Can you work these out from the drawing? Everything is in mm from the part's minimum corner. A direction names the side the tool comes from. Coordinates: 2 decimals unless noted, no trailing zeros. Order: outer loops, then holes, each group sorted by start corner. A loop starts at its lowest first (then second) coordinate and runs counter-clockwise, first axis right, second up. Notation, with made-up numbers: (84, 62) - (126, 62) arc R23 ccw to (126, 79) - close; hole circle Ø2 at (13.25, 88). An arc over 180 degrees is marked (long way). Answer as CSV lines item,"result". Start each with the question number.
Item 1: I'm going to push flat-ended pins straight in: pin 1 (2 mm diameter, centred on y = 9.5, z = 15, fed in from +X); pin 2 (4 mm diameter, centred on x = 11.5, y = 3.5, fed in from +Z); pin 3 (5 mm diameter, centred on x = 13, z = 3, fed in from +Y). Where does each tip first touch, or does it pass through?
Item 2: Imagine slicing it at B-B on z = 9.25. List the corners of the cut face in (x, y) for me.
Item 3: We'd pull the mould along X, two halves only. Please class the marked faces 6, 7 and 8: pulls with the +X half, pulls with the -X half, needs draft (parallel to the pull), parting line crosses it, or undercut.
Item 4: Imagine slicing it at D-D on y = 8. List the corners of the cut face in (x, z) for me, and give its area (3 significant figures).
Item 5: On a 3-axis mill with a long thin cutter (end or side, diameter ignored), from which of +Z, -Z, +X, -X, +Y, -Y can I reach the whole of each face in a straight line? I mean the marked faces 1, 2, 3, 4 and 5. Say none if no direction works.
Item 6: I need wall thicknesses on line 1 (X direction, y = 12.75, z = 8.5); line 2 (Z direction, x = 22.25, y = 1.75). Which ranges of each line are inside material? Lowest first, please.
Item 7: Imagine slicing it at C-C on x = 14. List the corners of the cut face in (y, z) for me, and give its area (3 significant figures).
Item 8: Imagine slicing it at A-A on y = 15. List the corners of the cut face in (x, z) for me, and give its area (3 significant figures).
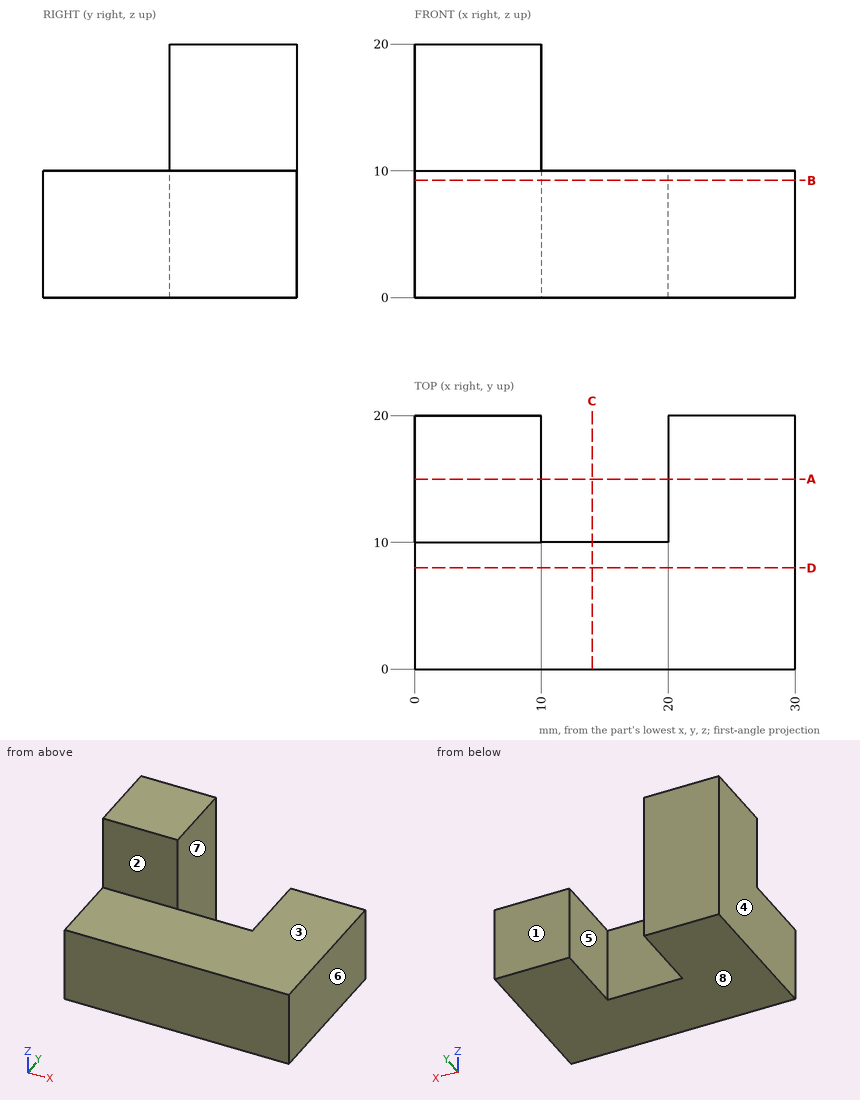
Responses:
1,pin 1,"stops at x = 10"
1,pin 2,"stops at z = 10"
1,pin 3,"stops at y = 10"
2,outline,"(0, 0) - (30, 0) - (30, 20) - (20, 20) - (20, 10) - (10, 10) - (10, 20) - (0, 20) - close"
3,face 6,"pulls with the +X half"
3,face 7,"undercut"
3,face 8,"needs draft"
4,outline,"(0, 0) - (30, 0) - (30, 10) - (0, 10) - close"
4,area,"300 mm^2"
5,face 1,"+Z, -Z, +X, -X, +Y"
5,face 2,"+Z, +X, -X, -Y"
5,face 3,"+Z, +X, -Y"
5,face 4,"+Z, -Z, -X, +Y, -Y"
5,face 5,"+Z, -Z, +Y"
6,line 1,"x = 0 to 10, 20 to 30"
6,line 2,"z = 0 to 10"
7,outline,"(0, 0) - (10, 0) - (10, 10) - (0, 10) - close"
7,area,"100 mm^2"
8,outline,"(0, 0) - (10, 0) - (10, 20) - (0, 20) - close; (20, 0) - (30, 0) - (30, 10) - (20, 10) - close"
8,area,"300 mm^2"
